Check sheet for the modelled part. Datum: model origin and axes. Units: mm. Round coordinates to 2 decimals unless told otherwise and drop trailing zeros. Write each loop counter-clockwise with the first axis right and the second up, starting at its lowest first coordinate (ties: lowest second). Pieces come first, ordered by that corner, then holes. Notation, with made-up numbers: (84, 82) - (107, 82) arc R21 ccw to (107, 96) - close; hole circle Ø9 at (12.5, -13.5). An arc over 180 degrees is marked (long way). Answer as a JSON object with one key per item and string values. Group by question number.
Item 1: Sectioned sample at B-B on z = 44.5. Record the boundary of the cut face in (x, y), plus the area to 3 significant figures.
Item 2: Thickness scan on line 1 (Z direction, x = 0.5, y = 0.5); line 2 (Z direction, x = -5, y = 1.75); line 3 (Z direction, x = 2.25, y = 4.5). Record the ranges inside material, lowest first.
Item 3: Release check for a two-part mould opening along Z. For faces 1 (the cylindrical face through (-0.018, -4.822, 201.751)), 2 (the cylindrical face through (0.089, -0.688, 191.846)), 3 (the flat face through (0, 0, 0)) record: pulls with the +Z half, pulls with the -Z half, needs draft (parallel to the pull), parting line crosses it, or undercut.
```python
from build123d import *

# Parameters (mm, degrees)
F0_W         = 12.7
F0_H         = 12.7
F1_DEPTH     = 203.2
F2_R         = 3.175
F3_DEPTH     = 25.4
F4_T1_DEPTH  = 210.82
F4_T3_DEPTH  = 2.54
F4_T5_DEPTH  = 2.54
F4_S9_W      = 5.08
F4_S9_H      = 5.08
F4_T10_DEPTH = 5.08
F4_S15_W     = 5.08
F4_S15_H     = 5.08
F4_T16_DEPTH = 5.08
F4_S21_W     = 5.08
F4_S21_H     = 5.08
F4_T22_DEPTH = 5.08
F4_S27_W     = 5.08
F4_S27_H     = 5.08
F4_T28_DEPTH = 5.08


# Not quite as in the source:
# - a fillet or chamfer that OpenCascade refuses, or shapes differently, is made with other operations: its cross-section is extruded or revolved along the edge and cut away or added


with BuildPart() as f1:
    # F0 (on Top) → F1 (new body)
    with BuildSketch(Plane.XY):
        Rectangle(F0_W, F0_H)
    extrude(amount=F1_DEPTH)

    # F2 (on face) → F3 (cut)
    with BuildSketch(Plane.YZ.offset(6.35)):
        with Locations((0, 194.945)):
            Circle(F2_R)
    extrude(amount=-F3_DEPTH, mode=Mode.SUBTRACT)

    # F4: fillet of radius 5.08 on 8 edges, made by hand

    # F4_s2 → F4_t1 (cut)
    with BuildSketch(Plane.XY.offset(-12.7)):
        with BuildLine():
            ThreePointArc((1.27, 6.35), (4.8621024484, 4.8621024484), (6.35, 1.27))
            Line((6.35, 1.27), (6.35, 6.35))
            Line((6.35, 6.35), (1.27, 6.35))
        make_face()
        with BuildLine():
            ThreePointArc((6.35, -1.27), (4.8621024484, -4.8621024484), (1.27, -6.35))
            Line((1.27, -6.35), (6.35, -6.35))
            Line((6.35, -6.35), (6.35, -1.27))
        make_face()
        with BuildLine():
            ThreePointArc((-1.27, 6.35), (-4.8621024484, 4.8621024484), (-6.35, 1.27))
            Line((-6.35, 1.27), (-6.35, 6.35))
            Line((-6.35, 6.35), (-1.27, 6.35))
        make_face()
        with BuildLine():
            ThreePointArc((-6.35, -1.27), (-4.8621024484, -4.8621024484), (-1.27, -6.35))
            Line((-1.27, -6.35), (-6.35, -6.35))
            Line((-6.35, -6.35), (-6.35, -1.27))
        make_face()
    extrude(amount=F4_T1_DEPTH, mode=Mode.SUBTRACT)

    # F4_s4 → F4_t3 (cut)
    with BuildSketch(Plane.YZ.offset(-1.27)):
        with BuildLine():
            ThreePointArc((6.35, 198.12), (4.8621024484, 201.7121024484), (1.27, 203.2))
            Line((1.27, 203.2), (6.35, 203.2))
            Line((6.35, 203.2), (6.35, 198.12))
        make_face()
        with BuildLine():
            ThreePointArc((-1.27, 203.2), (-4.8621024484, 201.7121024484), (-6.35, 198.12))
            Line((-6.35, 198.12), (-6.35, 203.2))
            Line((-6.35, 203.2), (-1.27, 203.2))
        make_face()
    extrude(amount=F4_T3_DEPTH, mode=Mode.SUBTRACT)

    # F4_s6 → F4_t5 (cut)
    with BuildSketch(Plane.XZ.offset(-1.27)):
        with BuildLine():
            ThreePointArc((6.35, 198.12), (4.8621024484, 201.7121024484), (1.27, 203.2))
            Line((1.27, 203.2), (6.35, 203.2))
            Line((6.35, 203.2), (6.35, 198.12))
        make_face()
        with BuildLine():
            ThreePointArc((-6.35, 198.12), (-4.8621024484, 201.7121024484), (-1.27, 203.2))
            Line((-1.27, 203.2), (-6.35, 203.2))
            Line((-6.35, 203.2), (-6.35, 198.12))
        make_face()
    extrude(amount=F4_T5_DEPTH, mode=Mode.SUBTRACT)


with BuildPart() as f4_tool8:
    # F4_s9 → F4_t10 (new body)
    with BuildSketch(Plane.XZ.offset(-1.27)):
        with Locations((3.81, 200.66)):
            Rectangle(F4_S9_W, F4_S9_H)
    extrude(amount=-F4_T10_DEPTH)

    # F4_s11 → F4_t12 (revolve, cut)
    with BuildSketch(Plane(origin=(1.27, 1.27, 198.12), x_dir=(-0.7071067812, 0, -0.7071067812), z_dir=(0.7071067812, 0, -0.7071067812))):
        with BuildLine():
            ThreePointArc((0, -5.08), (5.08, 0), (0, 5.08))
            Line((0, 5.08), (0, -5.08))
        make_face()
    revolve(axis=Axis((1.27, 1.27, 198.12), (0, 1, 0)), mode=Mode.SUBTRACT)


with BuildPart() as f1_1:
    add(f1.part)

    # F4_t7: cut F4_tool8
    add(f4_tool8.part, mode=Mode.SUBTRACT)


with BuildPart() as f4_tool14:
    # F4_s15 → F4_t16 (new body)
    with BuildSketch(Plane.YZ.offset(1.27)):
        with Locations((-3.81, 200.66)):
            Rectangle(F4_S15_W, F4_S15_H)
    extrude(amount=F4_T16_DEPTH)

    # F4_s17 → F4_t18 (revolve, cut)
    with BuildSketch(Plane(origin=(1.27, -1.27, 198.12), x_dir=(0, 0.7071067812, -0.7071067812), z_dir=(0, -0.7071067812, -0.7071067812))):
        with BuildLine():
            ThreePointArc((0, -5.08), (5.08, 0), (0, 5.08))
            Line((0, 5.08), (0, -5.08))
        make_face()
    revolve(axis=Axis((1.27, -1.27, 198.12), (1, 0, 0)), mode=Mode.SUBTRACT)


with BuildPart() as f1_2:
    add(f1_1.part)

    # F4_t13: cut F4_tool14
    add(f4_tool14.part, mode=Mode.SUBTRACT)


with BuildPart() as f4_tool20:
    # F4_s21 → F4_t22 (new body)
    with BuildSketch(Plane.XZ.offset(-1.27)):
        with Locations((-3.81, 200.66)):
            Rectangle(F4_S21_W, F4_S21_H)
    extrude(amount=-F4_T22_DEPTH)

    # F4_s23 → F4_t24 (revolve, cut)
    with BuildSketch(Plane(origin=(-1.27, 1.27, 198.12), x_dir=(0.7071067812, 0, -0.7071067812), z_dir=(0.7071067812, 0, 0.7071067812))):
        with BuildLine():
            ThreePointArc((0, -5.08), (5.08, 0), (0, 5.08))
            Line((0, 5.08), (0, -5.08))
        make_face()
    revolve(axis=Axis((-1.27, 1.27, 198.12), (0, 1, 0)), mode=Mode.SUBTRACT)


with BuildPart() as f1_3:
    add(f1_2.part)

    # F4_t19: cut F4_tool20
    add(f4_tool20.part, mode=Mode.SUBTRACT)


with BuildPart() as f4_tool26:
    # F4_s27 → F4_t28 (new body)
    with BuildSketch(Plane.YZ.offset(-1.27)):
        with Locations((-3.81, 200.66)):
            Rectangle(F4_S27_W, F4_S27_H)
    extrude(amount=-F4_T28_DEPTH)

    # F4_s29 → F4_t30 (revolve, cut)
    with BuildSketch(Plane(origin=(-1.27, -1.27, 198.12), x_dir=(0, 0.7071067812, -0.7071067812), z_dir=(0, 0.7071067812, 0.7071067812))):
        with BuildLine():
            ThreePointArc((0, -5.08), (5.08, 0), (0, 5.08))
            Line((0, 5.08), (0, -5.08))
        make_face()
    revolve(axis=Axis((-1.27, -1.27, 198.12), (-1, 0, 0)), mode=Mode.SUBTRACT)


with BuildPart() as f1_4:
    add(f1_3.part)

    # F4_t25: cut F4_tool26
    add(f4_tool26.part, mode=Mode.SUBTRACT)


solid = f1_4.part
```
Completed:
{
 "1": {"outline": "(-6.35, -1.27) arc R5.08 ccw to (-1.27, -6.35) - (1.27, -6.35) arc R5.08 ccw to (6.35, -1.27) - (6.35, 1.27) arc R5.08 ccw to (1.27, 6.35) - (-1.27, 6.35) arc R5.08 ccw to (-6.35, 1.27) - close", "area": "139 mm²"},
 "2": {"line 1": "0 to 191.81, 198.08 to 203.2", "line 2": "0 to 192.3, 197.59 to 201.54", "line 3": "0 to 201.92"},
 "3": {"face 1": "pulls with the +Z half", "face 2": "undercut", "face 3": "pulls with the -Z half"}
}
